Geometry: final body of the model. Coordinates: model frame, mm. A direction names the side the tool comes from. Round coordinates to 2 decimals unless told otherwise and drop trailing zeros. Write each loop counter-clockwise with the first axis right and the second up, starting at its lowest first coordinate (ties: lowest second). Pieces come first, ordered by that corner, then holes. Notation, with made-up numbers: (68, -28.5) - (116, -28.5) arc R25 cw to (116, -1.5) - close; hole circle Ø2 at (27.5, -32.75). An arc over 180 degrees is marked (long way). Use a Markdown table: item, result. Add a question column.
```python
from build123d import *

# Parameters (mm, degrees)
F0_R     = 1.15
F0_R_2   = 1.25
F1_DEPTH = 1.6
F2_W     = 7.6
F2_H     = 7.9
F3_DEPTH = 5.5
F4_W     = 8.09
F4_H     = 0.28
F4_H_2   = 5.32
F5_DEPTH = 2.45


with BuildPart() as f1:
    # F0 (on Top) → F1 (new body)
    with BuildSketch(Plane.XY):
        with BuildLine():
            ThreePointArc((10.795, 15.24), (10.051051, 17.036051), (8.255, 17.78))
            Line((8.255, 17.78), (-8.255, 17.78))
            ThreePointArc((-8.255, 17.78), (-10.051051, 17.036051), (-10.795, 15.24))
            Line((-10.795, 15.24), (-10.795, -15.24))
            ThreePointArc((-10.795, -15.24), (-10.051051, -17.036051), (-8.255, -17.78))
            Line((-8.255, -17.78), (8.255, -17.78))
            ThreePointArc((8.255, -17.78), (10.051051, -17.036051), (10.795, -15.24))
            Line((10.795, -15.24), (10.795, 15.24))
        make_face()
        with Locations((-6.575, -15.49)):
            Circle(F0_R, mode=Mode.SUBTRACT)
        with Locations((6.575, -15.49)):
            Circle(F0_R, mode=Mode.SUBTRACT)
        with Locations((-8.255, 15.24)):
            Circle(F0_R_2, mode=Mode.SUBTRACT)
        with Locations((8.255, 15.24)):
            Circle(F0_R_2, mode=Mode.SUBTRACT)
    extrude(amount=-F1_DEPTH)

    # F2 (on Top) → F3 (join)
    with BuildSketch(Plane.XY):
        with Locations((-7.135, 5.54)):
            Rectangle(F2_W, F2_H)
    extrude(amount=F3_DEPTH)

    # F4 (on face) → F5 (join)
    with BuildSketch(Plane.XY):
        with Locations((0.06, 17.92)):
            Rectangle(F4_W, F4_H)
        with Locations((0.06, 15.12)):
            Rectangle(F4_W, F4_H_2)
    extrude(amount=F5_DEPTH)


solid = f1.part
```
1) Section B-B, the plane x = 1. Return the cut outline in (y, z).
2) Pin query (flat end, axial travel): P1, Ø1.6, axis at x = -8, z = 3.5, coming from the +Y side; P2, Ø1.6, axis at y = 4, z = 2.5, coming from the +X side (3 decimals); P3, Ø3, axis at x = -7, y = -13, coming from the +Z side. Return the tip coordinate at first contact, or that it passes through.
3) Draft query along X for faces 1 (the cylindrical face through (-6.824, -16.613, -0.789)), 2 (the flat face through (0, -17.78, -1)), 3 (the flat face through (-10.795, 0, -1)). Return one class per face: released by +X, released by -X, zero draft, split by the parting line, or undercut.
4) Section C-C, the plane y = 3. Return the cut outline in (x, z) (3 decimals).
5) Set-up query: faces 4 (the flat face through (-7, 1.59, 3)), 5 (the cylindrical face through (5.662, -16.19, -0.789)), 6 (the flat face through (-3.335, 5, 3)), 7 (the flat face through (4.105, 15, 1)). Return all of +Z, -Z, +X, -X, +Y, -Y with unobstructed straight access to the full face (end or side cutting, diameter ignored); none if empty.
6) Section A-A, the plane z = 0.75. Return the cut outline in (x, y) (3 decimals).
7) Material intervals for L1, parallel to Y at x = -9.25, z = 3; L2, parallel to Z at x = -1.5, y = 5; L3, parallel to Y at x = -1.5, z = 0.25, sorted ascending. Write a range as from..to.
Output values:
| question | item | result |
|---|---|---|
| 1 | outline | (-17.78, -1.6) - (17.78, -1.6) - (17.78, 0) - (18.06, 0) - (18.06, 2.45) - (12.46, 2.45) - (12.46, 0) - (-17.78, 0) - close |
| 2 | P1 | stops at y = 9.49 |
| 2 | P2 | stops at x = -3.335 |
| 2 | P3 | stops at z = 0 |
| 3 | face 1 | undercut |
| 3 | face 2 | zero draft |
| 3 | face 3 | released by -X |
| 4 | outline | (-10.935, 0) - (-10.795, 0) - (-10.795, -1.6) - (10.795, -1.6) - (10.795, 0) - (-3.335, 0) - (-3.335, 5.5) - (-10.935, 5.5) - close |
| 5 | face 4 | +Z, +X, -X, -Y |
| 5 | face 5 | +Z, -Z |
| 5 | face 6 | +Z, +X, -Y |
| 5 | face 7 | +Z, +X, +Y, -Y |
| 6 | outline | (-10.935, 1.59) - (-3.335, 1.59) - (-3.335, 9.49) - (-10.935, 9.49) - close; (-3.985, 12.46) - (4.105, 12.46) - (4.105, 18.06) - (-3.985, 18.06) - close |
| 7 | L1 | y = 1.59..9.49 |
| 7 | L2 | z = -1.6..0 |
| 7 | L3 | y = 12.46..18.06 |
